Part model, mm, in its own coordinate system. Coordinates: 2 decimals unless noted, no trailing zeros. Order: outer loops, then holes, each group sorted by start corner. A loop starts at its lowest first (then second) coordinate and runs counter-clockwise, first axis right, second up.
1) Cut at A-A (z = 23.5). List the corners of the cut face in (x, y), and give its area (3 significant figures).
2) Wall check: L1, parallel to Y at x = -51.75, z = 68; L2, parallel to Y at x = -61, z = 57; L3, parallel to Z at x = -46.5, y = 58.75. Give the ranges that are in metal, low to high.
3) Pin check, flat tips, straight feed: pin 1 Ø8 at (y, z) = (63.5, 18.5) entering from +X; pin 2 Ø1.5 at (x, y) = (-54.5, 46) entering from +Z; pin 3 Ø8 at (y, z) = (46.5, 36) entering from +X. Stop position of each tip, or through.
```python
from build123d import *

# Parameters (mm, degrees)
F0_R     = 12.7
F1_DEPTH = 76.2
F2_SIZE  = 7.62
F3_SIZE  = 7.62


with BuildPart() as f1:
    # F0 (on Top) → F1 (new body)
    with BuildSketch(Plane.XY):
        with Locations((-52.293554, 54.482132)):
            Circle(F0_R)
    extrude(amount=F1_DEPTH)

    # F2
    f2_edges = [f1.edges().sort_by_distance(p)[0] for p in [
        (-64.993554, 54.482132, 76.2),
    ]]
    chamfer(f2_edges, length=F2_SIZE)

    # F3
    f3_edges = [f1.edges().sort_by_distance(p)[0] for p in [
        (-64.993554, 54.482132, 0),
    ]]
    chamfer(f3_edges, length=F3_SIZE)


solid = f1.part
```
Geometry check:
1. outline: circle Ø25.4 at (-52.29, 54.48)
1. area: 507 mm2
2. L1: y = 41.79 to 67.17
2. L2: y = 45.24 to 63.73
2. L3: z = 2.12 to 74.08
3. pin 1: stops at x = -40.63
3. pin 2: stops at z = 73.27
3. pin 3: stops at x = -40.23
